```python
from build123d import *

# Parameters (mm, degrees)
SKETCH_1_R               = 4
SKETCH_1_R_2             = 2.5
EXTRUDE_1_DEPTH          = 100
CUT_EXTRUDE_1_DEPTH      = 101.159872204
CUT_EXTRUDE_1_DEPTH_BACK = 101.159872204
SKETCH_2_W               = 8
SKETCH_2_H               = 60


with BuildPart() as part:
    # 草图1 → 凸台-拉伸1 (new body)
    with BuildSketch(Plane(origin=(0, 0, 0), x_dir=(1, 0, 0), z_dir=(0, 1, 0))):
        with Locations(Location((0, 0, 0), (0, 0, 270))):
            Circle(SKETCH_1_R)
        with Locations(Location((0, 0, 0), (0, 0, 270))):
            Circle(SKETCH_1_R_2, mode=Mode.SUBTRACT)
    extrude(amount=EXTRUDE_1_DEPTH)

    # 草图2 → 切除-拉伸1 (cut, two sides: drawn at the far end of the back side and taken through both)
    with BuildSketch(Plane(origin=(0, 0, 0), x_dir=(0, 0, -1), z_dir=(1, 0, 0)).offset(-CUT_EXTRUDE_1_DEPTH_BACK)):
        with Locations((4, 50)):
            Rectangle(SKETCH_2_W, SKETCH_2_H)
    extrude(amount=CUT_EXTRUDE_1_DEPTH + CUT_EXTRUDE_1_DEPTH_BACK, mode=Mode.SUBTRACT)


solid = part.part
```
Build history of the part. All positions in model axes, mm. Give positions to 0.01 mm unless a question says otherwise; leave off trailing zeros. Loops run counter-clockwise (first coordinate to the right, second up) from the corner with the lowest first, then second, coordinate; pieces in that order, holes last.
Item 1: Pull direction Y, two halves, no side cores. Call faces 1 (the face through (0, 20, -3)), 2 (the face through (2, 100, 2)), 3 (the face through (0, 80, -3)), 4 (the face through (-1.532, 49.3, 3.695)): released by +Y, released by -Y, zero draft, split by the parting line, or undercut.
Answers follow:
face 1: undercut
face 2: released by +Y
face 3: undercut
face 4: zero draft
Item 2: Slice it at C-C, the plane z = 1. List the corners of the cut face in (x, y).
Answers follow:
outline: (-3.87, 0) - (-2.29, 0) - (-2.29, 100) - (-3.87, 100) - close; (2.29, 0) - (3.87, 0) - (3.87, 100) - (2.29, 100) - close
Item 3: Slice it at A-A, the plane x = 0. List the corners of the cut face in (y, z).
Answers follow:
outline: (0, -4) - (20, -4) - (20, -2.5) - (0, -2.5) - close; (0, 2.5) - (100, 2.5) - (100, 4) - (0, 4) - close; (80, -4) - (100, -4) - (100, -2.5) - (80, -2.5) - close
Item 4: Drill centre lines: line 1 (Y direction, x = 1, z = -2.5); line 2 (Z direction, x = 0, y = 68); line 3 (X direction, y = 76, z = 1.75). Where is each one in solid material? Low to high.
Answers follow:
line 1: y = 0 to 20, 80 to 100
line 2: z = 2.5 to 4
line 3: x = -3.6 to -1.79, 1.79 to 3.6
Item 5: Flat gauge pins, fed straight in: pin 1 (1.5 mm diameter, centred on y = 85.5, z = -3, fed in from -X); pin 2 (1.2 mm diameter, centred on x = 3.5, y = 50, fed in from -Z); pin 3 (1.5 mm diameter, centred on x = 1.5, y = 43, fed in from -Z). Where does each tip first touch, or does it go through?
Answers follow:
pin 1: stops at x = -3.31
pin 2: stops at z = 0
pin 3: stops at z = 1.09
Item 6: Slice it at D-D, the plane y = 53. List the corners of the cut face in (x, z).
Answers follow:
outline: (-4, 0) - (-2.5, 0) arc R2.5 cw to (2.5, 0) - (4, 0) arc R4 ccw to start
Item 7: Slice it at B-B, the plane y = 88. List the corners of the cut face in (x, z).
Answers follow:
outline: circle Ø8 at (0, 0); hole circle Ø5 at (0, 0)
